Design review of the part built by this model. Coordinates are the model's own, in mm. Face numbers are marked on the shaded views. A direction names the side the tool comes from. Round coordinates to 2 decimals unless told otherwise and drop trailing zeros. Loops run counter-clockwise (first coordinate to the right, second up) from the corner with the lowest first, then second, coordinate; pieces in that order, holes last. Notation, with made-up numbers: (59.25, -24) - (116.25, -24) arc R21 ccw to (116.25, -13) - close; hole circle Ø10 at (83.5, 12). An arc over 180 degrees is marked (long way). Answer as CSV lines item,"result". Start each with the question number.
(1) For the marked faces 4, 5, 6 and 7, list the 3-axis set-ups (+Z, -Z, +X, -X, +Y, -Y) from which the entire face can be reached by the end or side of a thin tool; tool diameter is ignored.
(2) Consider section C-C (x = 0). Give the boundary of the cut face in (y, z), and give its area (3 significant figures).
(3) Mouldability with a two-part tool opening along Z and no side actions: class the marked faces 1, 2 and 3 as released by +Z, released by -Z, zero draft, split by the parting line, or undercut.
(4) Consider section D-D (z = 29). Give the boundary of the cut face in (x, y).
(5) For P1, Ø4, axis at x = 1, z = -4, coming from the -Y side; P2, Ø1.8, axis at y = -7, z = 18.5, coming from the -X side; P3, Ø14.5, axis at x = -2, z = 26.5, coming from the -Y side; P4, Ø3, axis at y = -6.5, z = 18, coming from the +X side, all flat-tipped, find the tip position at first contact; note any pin that passes through.
(6) Consider section B-B (y = 8). Give the boundary of the cut face in (x, z).
(7) Wall thickness on L1, parallel to Z at x = 0, y = -7; L2, parallel to Y at x = -4.5, z = 19; L3, parallel to X at y = -1, z = -26: over which ranges is each line inside the solid? List them lowest first.
(8) Consider section A-A (z = 0). Give the boundary of the cut face in (x, y).
from build123d import *

# Parameters (mm, degrees)
BOSS_EXTRUDE1_DEPTH     = 23
BOSS_EXTRUDE3_DEPTH     = 11
BOSS_EXTRUDE4_START     = 5
SKETCH1_5_R             = 7
SKETCH1_5_R_2           = 5
BOSS_EXTRUDE4_DEPTH     = 6
BOSS_EXTRUDE5_START     = -11
SKETCH1_6_R             = 7
SKETCH1_6_R_2           = 5
BOSS_EXTRUDE5_DEPTH     = 6
BOSS_EXTRUDE6_DEPTH     = 9
FILLET5_RADIUS          = 9
FILLET5_LENGTH          = 6
FILLET6_RADIUS          = 9
FILLET6_LENGTH          = 6
CUT_EXTRUDE1_DEPTH      = 54.714523176
CUT_EXTRUDE1_DEPTH_BACK = 54.714523176
SKETCH3_R               = 5


with BuildPart() as part:
    # Sketch1 → Boss-Extrude1 (new, symmetric)
    with BuildSketch(Plane(origin=(0, 0, 0), x_dir=(0, 0, -1), z_dir=(1, 0, 0))):
        with BuildLine():
            Line((-17.656443583, 3.5), (-12.519984026, 3.5))
            ThreePointArc((-12.519984026, 3.5), (1.766381565, 12.879436951), (13, 0))
            ThreePointArc((13, 0), (1.766381565, -12.879436951), (-12.519984026, -3.5))
            Line((-12.519984026, -3.5), (-17.656443583, -3.5))
            ThreePointArc((-17.656443583, -3.5), (-16.743615691, -6.606915588), (-15.288884851, -9.5))
            ThreePointArc((-15.288884851, -9.5), (-5.96013191, -16.984605607), (6, -16.970562748))
            ThreePointArc((6, -16.970562748), (14.696938457, -10.392304845), (18, 0))
            ThreePointArc((18, 0), (14.696938457, 10.392304845), (6, 16.970562748))
            ThreePointArc((6, 16.970562748), (-5.96013191, 16.984605607), (-15.288884851, 9.5))
            ThreePointArc((-15.288884851, 9.5), (-16.743615691, 6.606915588), (-17.656443583, 3.5))
        make_face()
    extrude(amount=BOSS_EXTRUDE1_DEPTH, both=True)

    # Sketch1<4> → Boss-Extrude3 (add, symmetric)
    with BuildSketch(Plane(origin=(0, 0, 0), x_dir=(0, 0, -1), z_dir=(1, 0, 0))):
        with BuildLine():
            Line((21, 11.66726189), (6, 16.970562748))
            ThreePointArc((6, 16.970562748), (14.696938457, 10.392304845), (18, 0))
            ThreePointArc((18, 0), (14.696938457, -10.392304845), (6, -16.970562748))
            Line((6, -16.970562748), (21, -11.66726189))
            Line((21, -11.66726189), (21, 11.66726189))
        make_face()
    extrude(amount=BOSS_EXTRUDE3_DEPTH, both=True)

    # Sketch1<5> → Boss-Extrude4 (add)
    # profile 1 of 2: a face of its own
    with BuildSketch(Plane(origin=(0, 0, 0), x_dir=(0, 0, -1), z_dir=(1, 0, 0)).offset(BOSS_EXTRUDE4_START)):
        with BuildLine():
            Line((35.333333333, 6.599663291), (21, 11.66726189))
            Line((21, 11.66726189), (21, -11.66726189))
            Line((21, -11.66726189), (35.333333333, -6.599663291))
            ThreePointArc((35.333333333, -6.599663291), (26, 0), (35.333333333, 6.599663291))
        make_face()
    # profile 2 of 2: a face of its own
    with BuildSketch(Plane(origin=(0, 0, 0), x_dir=(0, 0, -1), z_dir=(1, 0, 0)).offset(BOSS_EXTRUDE4_START)):
        with Locations((33, 0)):
            Circle(SKETCH1_5_R)
        with Locations((33, 0)):
            Circle(SKETCH1_5_R_2, mode=Mode.SUBTRACT)
    extrude(amount=BOSS_EXTRUDE4_DEPTH)

    # Sketch1<6> → Boss-Extrude5 (add)
    # profile 1 of 2: a face of its own
    with BuildSketch(Plane(origin=(0, 0, 0), x_dir=(0, 0, -1), z_dir=(1, 0, 0)).offset(BOSS_EXTRUDE5_START)):
        with BuildLine():
            Line((35.333333333, 6.599663291), (21, 11.66726189))
            Line((21, 11.66726189), (21, -11.66726189))
            Line((21, -11.66726189), (35.333333333, -6.599663291))
            ThreePointArc((35.333333333, -6.599663291), (26, 0), (35.333333333, 6.599663291))
        make_face()
    # profile 2 of 2: a face of its own
    with BuildSketch(Plane(origin=(0, 0, 0), x_dir=(0, 0, -1), z_dir=(1, 0, 0)).offset(BOSS_EXTRUDE5_START)):
        with Locations((33, 0)):
            Circle(SKETCH1_6_R)
        with Locations((33, 0)):
            Circle(SKETCH1_6_R_2, mode=Mode.SUBTRACT)
    extrude(amount=BOSS_EXTRUDE5_DEPTH)

    # Sketch1<8> → Boss-Extrude6 (add, symmetric)
    with BuildSketch(Plane(origin=(0, 0, 0), x_dir=(0, 0, -1), z_dir=(1, 0, 0))):
        with BuildLine():
            Line((-35, 3.5), (-17.656443583, 3.5))
            ThreePointArc((-17.656443583, 3.5), (-16.743615691, 6.606915588), (-15.288884851, 9.5))
            Line((-15.288884851, 9.5), (-35, 9.5))
            Line((-35, 9.5), (-35, 3.5))
        make_face()
        with BuildLine():
            ThreePointArc((-15.288884851, -9.5), (-16.743615691, -6.606915588), (-17.656443583, -3.5))
            Line((-17.656443583, -3.5), (-35, -3.5))
            Line((-35, -3.5), (-35, -9.5))
            Line((-35, -9.5), (-15.288884851, -9.5))
        make_face()
    extrude(amount=BOSS_EXTRUDE6_DEPTH, both=True)

    # Fillet5: full round fillet: the end face becomes a half cylinder, R = half its width
    fillet5_face = Plane((0, 6.5, 35), x_dir=(0, 1, 0), z_dir=(0, 0, 1))  # on the end face: x along it, z out of the body
    fillet5_slab = fillet5_face.offset(-FILLET5_RADIUS / 2) * Box(FILLET5_LENGTH, 2 * FILLET5_RADIUS, FILLET5_RADIUS, mode=Mode.PRIVATE)  # the body's end, R deep
    fillet5_round = Plane((0, 6.5, 26), x_dir=(0, 0, 1), z_dir=(0, 1, 0)) * Cylinder(FILLET5_RADIUS, FILLET5_LENGTH, mode=Mode.PRIVATE)  # its axis R under the face
    add(fillet5_slab - fillet5_round, mode=Mode.SUBTRACT)

    # Fillet6: full round fillet: the end face becomes a half cylinder, R = half its width
    fillet6_face = Plane((0, -6.5, 35), x_dir=(0, -1, 0), z_dir=(0, 0, 1))  # on the end face: x along it, z out of the body
    fillet6_slab = fillet6_face.offset(-FILLET6_RADIUS / 2) * Box(FILLET6_LENGTH, 2 * FILLET6_RADIUS, FILLET6_RADIUS, mode=Mode.PRIVATE)  # the body's end, R deep
    fillet6_round = Plane((0, -6.5, 26), x_dir=(0, 0, 1), z_dir=(0, -1, 0)) * Cylinder(FILLET6_RADIUS, FILLET6_LENGTH, mode=Mode.PRIVATE)  # its axis R under the face
    add(fillet6_slab - fillet6_round, mode=Mode.SUBTRACT)

    # Sketch3 → Cut-Extrude1 (cut, two sides: drawn at the far end of the back side and taken through both)
    with BuildSketch(Plane(origin=(0, 9.5, 0), x_dir=(1, 0, 0), z_dir=(0, 1, 0)).offset(-CUT_EXTRUDE1_DEPTH_BACK)):
        with Locations(Location((0, -26, 0), (0, 0, 270))):
            Circle(SKETCH3_R)
    extrude(amount=CUT_EXTRUDE1_DEPTH + CUT_EXTRUDE1_DEPTH_BACK, mode=Mode.SUBTRACT)


solid = part.part
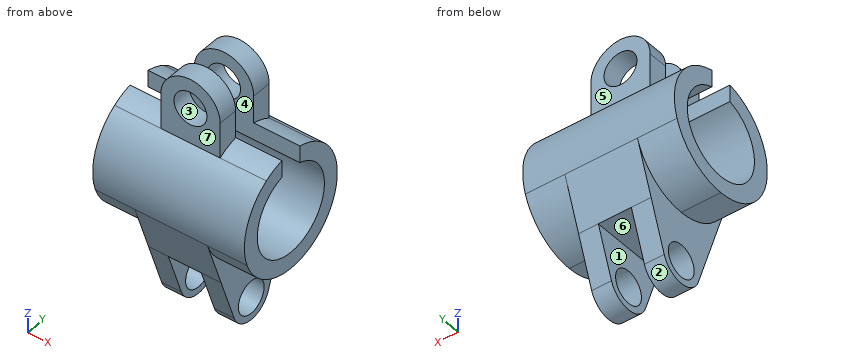
Determined:
1,face 4,"+Z, +X, -X"
1,face 5,"+Z, +X, -X, +Y"
1,face 6,"-Z, +Y, -Y"
1,face 7,"+Z, +X, -X, -Y"
2,outline,"(-16.97, -6) - (-11.67, -21) - (11.67, -21) - (16.97, -6) arc R18 ccw to (9.5, 15.29) - (9.5, 21) - (3.5, 21) - (3.5, 12.52) arc R13 cw (long way) to (-3.5, 12.52) - (-3.5, 21) - (-9.5, 21) - (-9.5, 15.29) arc R18 ccw to start; (-9.5, 31) - (-3.5, 31) - (-3.5, 35) - (-9.5, 35) - close; (3.5, 31) - (9.5, 31) - (9.5, 35) - (3.5, 35) - close"
2,area,"684 mm^2"
3,face 1,"zero draft"
3,face 2,"released by -Z"
3,face 3,"undercut"
4,outline,"(-8.49, -9.5) - (-4, -9.5) - (-4, -3.5) - (-8.49, -3.5) - close; (-8.49, 3.5) - (-4, 3.5) - (-4, 9.5) - (-8.49, 9.5) - close; (4, -9.5) - (8.49, -9.5) - (8.49, -3.5) - (4, -3.5) - close; (4, 3.5) - (8.49, 3.5) - (8.49, 9.5) - (4, 9.5) - close"
5,P1,"stops at y = -17.89"
5,P2,"stops at x = -9"
5,P3,"stops at y = -9.5"
5,P4,"stops at x = 23"
6,outline,"(-23, -16.12) - (-11, -16.12) - (-11, -31.37) - (-5, -31.37) - (-5, -21) - (5, -21) - (5, -31.37) - (11, -31.37) - (11, -16.12) - (23, -16.12) - (23, -10.25) - (-23, -10.25) - close; (-23, 10.25) - (23, 10.25) - (23, 16.12) - (9, 16.12) - (9, 26) arc R9 ccw to (-9, 26) - (-9, 16.12) - (-23, 16.12) - close; hole circle Ø10 at (0, 26)"
7,L1,"z = -21 to -10.95, 10.95 to 21, 31 to 35"
7,L2,"y = -9.5 to -3.5, 3.5 to 9.5"
7,L3,"x = -11 to -5, 5 to 11"
8,outline,"(-23, -18) - (23, -18) - (23, -13) - (-23, -13) - close; (-23, 13) - (23, 13) - (23, 18) - (-23, 18) - close"
